```python
from build123d import *

# Parameters (mm, degrees)
SKETCH_R        = 1.55
PAD_DEPTH       = 6.3
SKETCH002_W     = 5.6
SKETCH002_H     = 5.6
POCKET_DEPTH    = 2
PAD001_DEPTH    = 7.7
SKETCH003_R     = 1.65
POCKET001_DEPTH = 4.901
SKETCH004_W     = 5.6
SKETCH004_H     = 5.6
POCKET002_DEPTH = 2
SKETCH005_W     = 8
SKETCH005_H     = 7
PAD002_DEPTH    = 11.9
SKETCH006_R     = 1.6
PAD003_DEPTH    = 7.5
PAD004_DEPTH    = 11.9
SKETCH008_W     = 4.9
SKETCH008_H     = 22.3
PAD005_DEPTH    = 7
SKETCH009_R     = 1.65
POCKET003_DEPTH = 15.501
SKETCH010_W     = 5.6
SKETCH010_H     = 5.6
POCKET004_DEPTH = 2
CHAMFER_SIZE    = 7
FILLET_R        = 1.5
FILLET001_R     = 1


with BuildPart() as part:
    # Sketch → Pad (new body)
    with BuildSketch(Plane.YZ):
        Polygon((-4.9, -4.25), (0, -4.25), (0, -18.75), (-15, -18.75), (-15, -10.75), (-4.9, -10.75), align=None)
        with Locations((-11, -14.75)):
            Circle(SKETCH_R, mode=Mode.SUBTRACT)
        with Locations((-4, -14.75)):
            Circle(SKETCH_R, mode=Mode.SUBTRACT)
    extrude(amount=PAD_DEPTH)

    # Sketch002 (on Face9 of Pad) → Pocket (cut)
    with BuildSketch(Plane(origin=(0, 0, 0), x_dir=(0, 1, 0), z_dir=(-1, 0, 0))):
        with Locations((-4, 14.75)):
            Rectangle(SKETCH002_W, SKETCH002_H)
        with Locations((-11, 14.75)):
            Rectangle(SKETCH002_W, SKETCH002_H)
    extrude(amount=-POCKET_DEPTH, mode=Mode.SUBTRACT)

    # Sketch001 (on Face1 of Pad) → Pad001 (join)
    with BuildSketch(Plane(origin=(0, 0, -4.25), x_dir=(0, -1, 0), z_dir=(0, 0, 1))):
        Polygon((0, 0), (0, -16), (8, -16), (8, -9), (4.9, -9), (4.9, -2.7), (8, -2.7), (8, 0), align=None)
    extrude(amount=-PAD001_DEPTH)

    # Sketch003 (on Face1 of Pad001) → Pocket001 (cut, through all)
    with BuildSketch(Plane(origin=(0, -4.9, 0), x_dir=(0, 0, -1), z_dir=(0, -1, 0))):
        with Locations((7.9, -5.85)):
            Circle(SKETCH003_R)
        with Locations((7.9, 3.15)):
            Circle(SKETCH003_R)
    extrude(amount=-POCKET001_DEPTH, mode=Mode.SUBTRACT)

    # Sketch004 (on Face10 of Pocket001) → Pocket002 (cut)
    with BuildSketch(Plane.ZX):
        with Locations((-7.9, 3.15)):
            Rectangle(SKETCH004_W, SKETCH004_H)
        with Locations((-7.9, -5.85)):
            Rectangle(SKETCH004_W, SKETCH004_H)
    extrude(amount=-POCKET002_DEPTH, mode=Mode.SUBTRACT)

    # Sketch005 (on Face5 of Pocket002) → Pad002 (join)
    with BuildSketch(Plane(origin=(0, 0, -4.25), x_dir=(0, -1, 0), z_dir=(0, 0, 1))):
        with Locations((4, -12.5)):
            Rectangle(SKETCH005_W, SKETCH005_H)
    extrude(amount=PAD002_DEPTH)

    # Sketch006 (on Face36 of Pad002) → Pad003 (join)
    with BuildSketch(Plane(origin=(0, -8, 0), x_dir=(0, 0, -1), z_dir=(0, -1, 0))):
        with Locations((-2.25, -12.7)):
            Circle(SKETCH006_R)
        with Locations((2.25, -12.7)):
            Circle(SKETCH006_R)
    extrude(amount=PAD003_DEPTH)

    # Sketch007 (on Face7 of Pad003) → Pad004 (join)
    with BuildSketch(Plane(origin=(0, 0, -4.25), x_dir=(0, -1, 0), z_dir=(0, 0, 1))):
        Polygon((8, -2.5), (1.15, -2.5), (0, -1.35), (1.15, -0.2), (8, -0.2), align=None)
    extrude(amount=PAD004_DEPTH)

    # Sketch008 (on Face14 of Pad004) → Pad005 (join)
    with BuildSketch(Plane(origin=(0, 0, 7.65), x_dir=(0, -1, 0), z_dir=(0, 0, 1))):
        with Locations((2.45, -4.85)):
            Rectangle(SKETCH008_W, SKETCH008_H)
    extrude(amount=PAD005_DEPTH)

    # Sketch009 (on Face54 of Pad005) → Pocket003 (cut, through all)
    with BuildSketch(Plane.ZX):
        with Locations((11.1, 3.15)):
            Circle(SKETCH009_R)
        with Locations((11.1, -5.85)):
            Circle(SKETCH009_R)
    extrude(amount=-POCKET003_DEPTH, mode=Mode.SUBTRACT)

    # Sketch010 (on Face4 of Pocket003) → Pocket004 (cut)
    with BuildSketch(Plane.ZX):
        with Locations((11.1, 3.15)):
            Rectangle(SKETCH010_W, SKETCH010_H)
        with Locations((11.1, -5.85)):
            Rectangle(SKETCH010_W, SKETCH010_H)
    extrude(amount=-POCKET004_DEPTH, mode=Mode.SUBTRACT)

    # Chamfer
    chamfer_edges = [part.edges().sort_by_distance(p)[0] for p in [
        (-16, -2.45, 14.65),
        (-16, -4, -11.95),
    ]]
    chamfer(chamfer_edges, length=CHAMFER_SIZE)

    # Fillet
    fillet_edges = [part.edges().sort_by_distance(p)[0] for p in [
        (-12.5, -8, -8.45),
        (-16, -8, 1.35),
        (-12.5, -8, 7.65),
    ]]
    fillet(fillet_edges, radius=FILLET_R)

    # Fillet001
    fillet001_edges = [part.edges().sort_by_distance(p)[0] for p in [
        (-12.7, -15.5, -0.65),
        (-12.7, -15.5, 3.85),
    ]]
    fillet(fillet001_edges, radius=FILLET001_R)


solid = part.part
```
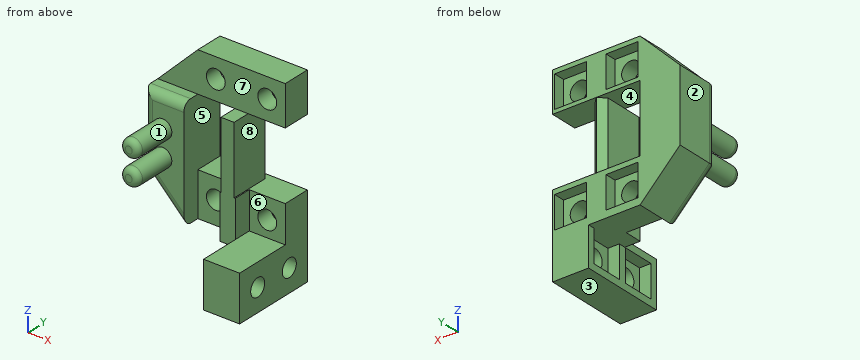
The model under review builds one solid part; all positions refer to its coordinate system, in mm. Face numbers are marked on the shaded views. A direction names the side the tool comes from. Round coordinates to 2 decimals unless told otherwise and drop trailing zeros. Loops run counter-clockwise (first coordinate to the right, second up) from the corner with the lowest first, then second, coordinate; pieces in that order, holes last. Notation, with made-up numbers: (-3.5, 65.5) - (4.5, 65.5) arc R24 ccw to (4.5, 82.5) - close; hole circle Ø6 at (2, -3). An arc over 180 degrees is marked (long way). Write each question's results on one line, items separated by ' | '. Start each with the question number.
Q1. Take a section at C-C on z = -14.75. Give the boundary of the cut face in (x, y).
Q2. Wall thickness on line 1 along Y through (x, z) = (3.45, -14.75); line 2 along X through (y, z) = (-3.2, 11.1); line 3 along Z through (x, y) = (5.4, -11): over which ranges is each line inside the solid? List them lowest first. Write a range as [from, to].
Q3. Tool access review of the marked faces 5, 6, 7 and 8: name each direction out of +Z, -Z, +X, -X, +Y, -Y from which nothing blocks a thin tool from reaching the whole face with its end or side.
Q4. Insertion check: P1, Ø1.6, axis at y = -1.5, z = -7, coming from the -X side; P2, Ø1.5, axis at y = -12.5, z = -1.5, coming from the +X side; P3, Ø1, axis at y = -0.5, z = -7.5, coming from the -X side. Each pin has a flat end and moves straight along its axis. Give the tip position at first contact, or say it passes through.
Q5. Take a section at A-A on y = -11. Give the boundary of the cut face in (x, z).
Q6. Take a section at D-D on x = -8. Give the boundary of the cut face in (y, z).
Q7. Take a section at B-B on x = 3.15. Give the boundary of the cut face in (y, z), plus the area to 3 significant figures.
Q8. Draft analysis for pull direction Z (two halves, no side actions). For the marked faces 1, 2, 3 and 4, state which applies: pulls with the +Z half, pulls with the -Z half, needs draft (parallel to the pull), parting line crosses it, or undercut.
Data:
1) outline: (0, -15) - (6.3, -15) - (6.3, -12.55) - (2, -12.55) - (2, -13.8) - (0, -13.8) - close; (0, -8.2) - (2, -8.2) - (2, -9.45) - (6.3, -9.45) - (6.3, -5.55) - (2, -5.55) - (2, -6.8) - (0, -6.8) - close; (0, -1.2) - (2, -1.2) - (2, -2.45) - (6.3, -2.45) - (6.3, 0) - (0, 0) - close
2) line 1: y = [-15, -12.55], [-9.45, -5.55], [-2.45, 0] | line 2: x = [-12.55, -7.5], [-4.2, 1.5], [4.8, 6.3] | line 3: z = [-18.75, -16.3], [-13.2, -10.75]
3) face 5: -Y | face 6: +Z, +X, -Y | face 7: +Z, +X, -X, -Y | face 8: +X, +Y, -Y
4) P1: stops at x = -14.75 | P2: stops at x = -11.1 | P3: stops at x = -13.95
5) outline: circle Ø3.2 at (-12.7, -2.25); circle Ø3.2 at (-12.7, 2.25); (0, -18.75) - (6.3, -18.75) - (6.3, -16.3) - (2, -16.3) - (2, -17.55) - (0, -17.55) - close; (0, -11.95) - (2, -11.95) - (2, -13.2) - (6.3, -13.2) - (6.3, -10.75) - (0, -10.75) - close
6) outline: (-4.9, -11.95) - (0, -11.95) - (0, -10.7) - (-2, -10.7) - (-2, -5.1) - (0, -5.1) - (0, -4.25) - (-4.9, -4.25) - close; (-4.9, 7.65) - (0, 7.65) - (0, 8.3) - (-2, 8.3) - (-2, 13.9) - (0, 13.9) - (0, 14.65) - (-4.9, 14.65) - close
7) outline: (-15, -18.75) - (0, -18.75) - (0, -10.7) - (-2, -10.7) - (-2, -9.55) - (-4.9, -9.55) - (-4.9, -10.75) - (-15, -10.75) - close; (-4.9, -6.25) - (-2, -6.25) - (-2, -5.1) - (0, -5.1) - (0, -4.25) - (-4.9, -4.25) - close; (-4.9, 7.65) - (0, 7.65) - (0, 8.3) - (-2, 8.3) - (-2, 9.45) - (-4.9, 9.45) - close; (-4.9, 12.75) - (-2, 12.75) - (-2, 13.9) - (0, 13.9) - (0, 14.65) - (-4.9, 14.65) - close; hole circle Ø3.1 at (-11, -14.75); hole circle Ø3.1 at (-4, -14.75) | area: 130 mm²
8) face 1: undercut | face 2: needs draft | face 3: pulls with the -Z half | face 4: undercut
